from build123d import *

# Parameters (mm, degrees)
SKETCH003_W     = 128.778
SKETCH003_H     = 67.818
SKETCH003_W_2   = 122.428
SKETCH003_H_2   = 61.468
PAD002_DEPTH    = 1.905
SKETCH004_W     = 128.778
SKETCH004_H     = 67.818
SKETCH004_W_2   = 125.222
SKETCH004_H_2   = 64.262
PAD003_DEPTH    = 40.64
SKETCH009_W     = 10.16
SKETCH009_H     = 1.778
SKETCH009_W_2   = 1.778
SKETCH009_H_2   = 10.16
PAD008_DEPTH    = 4.318
PAD009_DEPTH    = 10.16
PAD010_DEPTH    = 10.16
FILLET001_R     = 2.032
SKETCH013_W     = 0.762
SKETCH013_H     = 2.54
SKETCH013_W_2   = 2.54
SKETCH013_H_2   = 0.762
POCKET_DEPTH    = 12.7
SKETCH018_W     = 16.764
SKETCH018_H     = 11.176
POCKET002_DEPTH = 1.778
FILLET002_R     = 2.032


with BuildPart() as part:
    # Sketch003 → Pad002 (new body)
    with BuildSketch(Plane.XY.offset(8.636)):
        Rectangle(SKETCH003_W, SKETCH003_H)
        Rectangle(SKETCH003_W_2, SKETCH003_H_2, mode=Mode.SUBTRACT)
    extrude(amount=PAD002_DEPTH)

    # Sketch004 → Pad003 (new body)
    with BuildSketch(Plane(origin=(0, 0, 8.636), x_dir=(1, 0, 0), z_dir=(0, 0, -1))):
        Rectangle(SKETCH004_W, SKETCH004_H)
        Rectangle(SKETCH004_W_2, SKETCH004_H_2, mode=Mode.SUBTRACT)
    extrude(amount=PAD003_DEPTH)

    # Sketch009 → Pad008 (new body)
    with BuildSketch(Plane(origin=(0, 0, -32.004), x_dir=(1, 0, 0), z_dir=(0, 0, -1))):
        with Locations((0, 33.02)):
            Rectangle(SKETCH009_W, SKETCH009_H)
        with Locations((0, -33.02)):
            Rectangle(SKETCH009_W, SKETCH009_H)
        with Locations((-63.5, 0)):
            Rectangle(SKETCH009_W_2, SKETCH009_H_2)
        with Locations((63.5, 0)):
            Rectangle(SKETCH009_W_2, SKETCH009_H_2)
    extrude(amount=PAD008_DEPTH)

    # Sketch010 → Pad009 (new body)
    with BuildSketch(Plane(origin=(-5.08, 0, 8.636), x_dir=(0, -1, 0), z_dir=(-1, 0, 0))):
        Polygon((-32.131, -44.958), (-32.131, -43.688), (-31.115, -43.688), align=None)
        Polygon((32.131, -44.958), (32.131, -43.688), (31.115, -43.688), align=None)
    extrude(amount=-PAD009_DEPTH)

    # Sketch011 → Pad010 (new body)
    with BuildSketch(Plane(origin=(0, -5.08, 8.636), x_dir=(1, 0, 0), z_dir=(0, -1, 0))):
        Polygon((-62.611, -44.958), (-62.611, -43.688), (-61.595, -43.688), align=None)
        Polygon((62.611, -44.958), (62.611, -43.688), (61.595, -43.688), align=None)
    extrude(amount=-PAD010_DEPTH)

    # Fillet001
    fillet001_edges = [part.edges().sort_by_distance(p)[0] for p in [
        (64.389, -33.909, 9.5885),
        (64.389, -33.909, -11.684),
        (64.389, 33.909, 9.5885),
        (64.389, 33.909, -11.684),
        (-64.389, 33.909, -11.684),
        (-64.389, 33.909, 9.5885),
        (-64.389, -33.909, -11.684),
        (-64.389, -33.909, 9.5885),
    ]]
    fillet(fillet001_edges, radius=FILLET001_R)

    # Sketch013 → Pocket (cut)
    with BuildSketch(Plane(origin=(0, 0, -32.004), x_dir=(1, 0, 0), z_dir=(0, 0, -1))):
        with Locations((-5.461, 32.639)):
            Rectangle(SKETCH013_W, SKETCH013_H)
        with Locations((5.461, 32.639)):
            Rectangle(SKETCH013_W, SKETCH013_H)
        with Locations((-5.461, -32.639)):
            Rectangle(SKETCH013_W, SKETCH013_H)
        with Locations((5.461, -32.639)):
            Rectangle(SKETCH013_W, SKETCH013_H)
        with Locations((-63.119, 5.461)):
            Rectangle(SKETCH013_W_2, SKETCH013_H_2)
        with Locations((-63.119, -5.461)):
            Rectangle(SKETCH013_W_2, SKETCH013_H_2)
        with Locations((63.119, 5.461)):
            Rectangle(SKETCH013_W_2, SKETCH013_H_2)
        with Locations((63.119, -5.461)):
            Rectangle(SKETCH013_W_2, SKETCH013_H_2)
    extrude(amount=-POCKET_DEPTH, mode=Mode.SUBTRACT)

    # Sketch018 → Pocket002 (cut)
    with BuildSketch(Plane(origin=(0, 33.909, 8.636), x_dir=(-1, 0, 0), z_dir=(0, 1, 0))):
        with Locations((37.973, -35.052)):
            Rectangle(SKETCH018_W, SKETCH018_H)
    extrude(amount=-POCKET002_DEPTH, mode=Mode.SUBTRACT)

    # Fillet002
    fillet002_edges = [part.edges().sort_by_distance(p)[0] for p in [
        (-46.355, 33.02, -32.004),
        (-46.355, 33.02, -20.828),
        (-29.591, 33.02, -20.828),
        (-29.591, 33.02, -32.004),
    ]]
    fillet(fillet002_edges, radius=FILLET002_R)


solid = part.part
Design review of the part built by this model. Coordinates are the model's own, in mm. A direction names the side the tool comes from. Round coordinates to 2 decimals unless told otherwise and drop trailing zeros. Write each loop counter-clockwise with the first axis right and the second up, starting at its lowest first coordinate (ties: lowest second). Pieces come first, ordered by that corner, then holes. Notation, with made-up numbers: (49.5, 27.25) - (68.5, 27.25) arc R36 cw to (68.5, 62.25) - close; hole circle Ø8 at (59, -20). An arc over 180 degrees is marked (long way). Return JSON: item names as keys, results as strings. Group by question number.
Item 1: We need section C-C on z = -17. Write out the cut boundary in (x, y).
Item 2: For probe 1 along Y at (x, z) = (-5, -18); probe 2 along X at (y, z) = (18.5, 0.5); probe 3 along Z at (x, y) = (21, -31), list the stretches that pass through material, from the lowest coordinate up. Write a range as [from, to].
Item 3: We need section D-D on x = -17. Write out the cut boundary in (y, z), and give its area (3 significant figures).
Item 4: Insertion check: P1, Ø1.4, axis at y = -32, z = -26.5, coming from the -X side; P2, Ø0.9, axis at y = -32.5, z = -23.5, coming from the +X side; P3, Ø0.5, axis at x = -63.5, z = -27, coming from the -Y side; P4, Ø0.9, axis at x = 63.5, z = -25, coming from the +Y side. Each pin has a flat end and moves straight along its axis. Give the tip position at first contact, or say it passes through.
Item 5: The part is to be moulded in two halves that separate along Z. For faces 4 (the face through (-62.611, 0, -13)), 5 (the face through (62.611, 0, -13)), 6 (the face through (-43.9, -32.4, -32.004)), 7 (the face through (-5.08, 33, -28)), say which applies: pulls with the +Z half, pulls with the -Z half, needs draft (parallel to the pull), parting line crosses it, or undercut.
Item 6: We need section A-A on y = -3. Write out the cut boundary in (x, z) (3 decimals), and give its area (3 significant figures).
Item 7: We need section B-B on x = -1. Write out the cut boundary in (y, z) (3 decimals).
Item 8: Machinability: for faces 1 (the face through (5.08, -33, -28)), 2 (the face through (-1, -32.131, -13)), 3 (the face through (63, 5.08, -28)), which of the approach directions +Z, -Z, +X, -X, +Y, -Y give a long, thin tool a straight path to every point of the face, cutting with its end or side? Answer none if there is none.
Model answer:
{
 "1": {"outline": "(-64.39, -31.88) arc R2.03 ccw to (-62.36, -33.91) - (62.36, -33.91) arc R2.03 ccw to (64.39, -31.88) - (64.39, 31.88) arc R2.03 ccw to (62.36, 33.91) - (-62.36, 33.91) arc R2.03 ccw to (-64.39, 31.88) - close; hole (-62.61, -32.13) - (62.61, -32.13) - (62.61, 32.13) - (-62.61, 32.13) - close"},
 "2": {"probe 1": "y = [-33.91, -32.13], [32.13, 33.91]", "probe 2": "x = [-64.39, -62.61], [62.61, 64.39]", "probe 3": "z = [8.64, 10.54]"},
 "3": {"outline": "(-33.91, -32) - (-32.13, -32) - (-32.13, 8.64) - (-30.73, 8.64) - (-30.73, 10.54) - (-33.91, 10.54) - close; (30.73, 8.64) - (32.13, 8.64) - (32.13, -32) - (33.91, -32) - (33.91, 10.54) - (30.73, 10.54) - close", "area": "157 mm²"},
 "4": {"P1": "stops at x = -64.39", "P2": "stops at x = 64.38", "P3": "stops at y = -33.7", "P4": "stops at y = 33.79"},
 "5": {"face 4": "undercut", "face 5": "undercut", "face 6": "pulls with the -Z half", "face 7": "needs draft"},
 "6": {"outline": "(-64.389, -36.322) - (-62.611, -36.322) - (-61.595, -35.052) - (-62.611, -35.052) - (-62.611, 8.636) - (-61.214, 8.636) - (-61.214, 10.541) - (-64.389, 10.541) - close; (61.214, 8.636) - (62.611, 8.636) - (62.611, -35.052) - (61.595, -35.052) - (62.611, -36.322) - (64.389, -36.322) - (64.389, 10.541) - (61.214, 10.541) - close", "area": "173 mm²"},
 "7": {"outline": "(-33.909, -36.322) - (-32.131, -36.322) - (-31.115, -35.052) - (-32.131, -35.052) - (-32.131, 8.636) - (-30.734, 8.636) - (-30.734, 10.541) - (-33.909, 10.541) - close; (30.734, 8.636) - (32.131, 8.636) - (32.131, -35.052) - (31.115, -35.052) - (32.131, -36.322) - (33.909, -36.322) - (33.909, 10.541) - (30.734, 10.541) - close"},
 "8": {"face 1": "-Z, +Y, -Y", "face 2": "none", "face 3": "-Z, +X, -X"}
}
